Work out the finished part from the listing and answer in its coordinate system (mm). A direction names the side the tool comes from. Round coordinates to 2 decimals unless told otherwise and drop trailing zeros. Loops run counter-clockwise (first coordinate to the right, second up) from the corner with the lowest first, then second, coordinate; pieces in that order, holes last. Notation, with made-up numbers: (32.5, 81.5) - (79.5, 81.5) arc R19 cw to (79.5, 116.5) - close; hole circle Ø10 at (54.5, 34). An arc over 180 degrees is marked (long way). Use CSV: the item, a comma, the result in double quotes. Start each with the question number.
from build123d import *

# Parameters (mm, degrees)
ESQUISSE1_R                  = 4.15
BOSS_EXTRU_1_DEPTH           = 15
ENL_V_MAT_EXTRU_1_REACH      = 122
ENL_V_MAT_EXTRU_1_END_RADIUS = 4.15
ESQUISSE2_R                  = 4.15
ENL_V_MAT_EXTRU_2_DEPTH      = 7.5
TROU_TARAUD_M6X1_01_D        = 5


with BuildPart() as part:
    # Esquisse1 → Boss.-Extru.1 (new body)
    with BuildSketch(Plane(origin=(0, 0, 0), x_dir=(1, 0, 0), z_dir=(0, 1, 0))):
        with BuildLine():
            Line((25, 31.224989992), (25, 95))
            ThreePointArc((25, 95), (0, 120), (-25, 95))
            Line((-25, 95), (-25, 31.224989992))
            ThreePointArc((-25, 31.224989992), (0, 40), (25, 31.224989992))
        make_face()
        with Locations(Location((0, 95, 0), (0, 0, 270))):  # turned: the seam where the file's is
            Circle(ESQUISSE1_R, mode=Mode.SUBTRACT)
    extrude(amount=BOSS_EXTRU_1_DEPTH)

    # Enlèv. mat.-Extru.1: up to this cylinder (the profile starts outside it)
    enl_v_mat_extru_1_end = Plane(origin=(0, 7.5, -95), z_dir=(0, -1, 0)) * Cylinder(ENL_V_MAT_EXTRU_1_END_RADIUS, 253.3, mode=Mode.PRIVATE)
    # Esquisse2 → Enlèv. mat.-Extru.1 (cut, up to the surface)
    with BuildSketch(Plane.XY, mode=Mode.PRIVATE) as enl_v_mat_extru_1_sk1:
        with Locations((0, 7.5)):
            Circle(ESQUISSE2_R)
    enl_v_mat_extru_1_tool1 = extrude(enl_v_mat_extru_1_sk1.sketch, amount=-ENL_V_MAT_EXTRU_1_REACH, mode=Mode.PRIVATE) - enl_v_mat_extru_1_end
    add(enl_v_mat_extru_1_tool1.solids().sort_by_distance((0, 7.5, 0))[0], mode=Mode.SUBTRACT)

    # Esquisse3 → Enlèv. mat.-Extru.2 (cut)
    with BuildSketch(Plane(origin=(0, 15, 0), x_dir=(-1, 0, 0), z_dir=(0, 1, 0))):
        with BuildLine():
            Line((4.15, -95), (4.15, -86.15))
            ThreePointArc((4.15, -86.15), (0, -82), (-4.15, -86.15))
            Line((-4.15, -86.15), (-4.15, -95))
            ThreePointArc((-4.15, -95), (0, -99.15), (4.15, -95))
        make_face()
    extrude(amount=-ENL_V_MAT_EXTRU_2_DEPTH, mode=Mode.SUBTRACT)

    # Trou taraudé M6x1.01 (through all)
    with Locations(Plane.XZ):
        with Locations((17.5, -45), (-17.5, -45)):
            Hole(TROU_TARAUD_M6X1_01_D / 2)


solid = part.part
Item 1: Which of the six approach directions +Z, -Z, +X, -X, +Y, -Y give full straight-line access (tool end or side, diameter ignored) to faces 1 (the cylindrical face through (-0.9, 3.45, -60.87)), 2 (the flat face through (-4.15, 11, -91)), 3 (the cylindrical face through (0, 12, -40))?
Item 2: Find the intervals of material crossed by probe 1 along X at (y, z) = (6.5, -95); probe 2 along Z at (x, y) = (-17.5, 4); probe 3 along X at (y, z) = (8.5, -68), in increasing order. Write a range as [from, to].
Item 3: The mould has two halves that part along Z. Classify faces 4 (the cylindrical face through (-16, 8, -47)), 5 (the cylindrical face through (0.55, 7.395, -119.994)), 6 (the flat face through (4.15, 11, -91)), 7 (the flat face through (25, 7, -63)): pulls with the +Z half, pulls with the -Z half, needs draft (parallel to the pull), parting line crosses it, or undercut.
Item 4: A cutting plane is placed at A-A (z = -45). Determine the outline of the cut face in (x, y).
Item 5: A cutting plane is placed at D-D (y = 5). Determine the outline of the cut face in (x, z).
Item 6: A cutting plane is placed at C-C (y = 13.75). Determine the outline of the cut face in (x, z), plus the area to 3 significant figures.
Item 7: Each of these flat-tipped pins is pushed along its axis until it touches: pin 1 Ø2 at (x, y) = (15, 4) entering from -Z; pin 2 Ø8 at (x, y) = (-13, 10.5) entering from +Z; pin 3 Ø4 at (x, y) = (-18, 5.5) entering from -Z; pin 4 Ø8 at (x, z) = (-17.5, -45) entering from -Y. Where does it stop, or does it pass through?
Item 8: A cutting plane is placed at B-B (x = 0). Determine the outline of the cut face in (y, z).
Result sheet:
1,face 1,"+Z"
1,face 2,"+Y"
1,face 3,"+Z, +Y, -Y"
2,probe 1,"[-25, -4.15], [4.15, 25]"
2,probe 2,"[-112.85, -47.5], [-42.5, -35.97]"
2,probe 3,"[-25, -4.03], [4.03, 25]"
3,face 4,"undercut"
3,face 5,"pulls with the -Z half"
3,face 6,"undercut"
3,face 7,"needs draft"
4,outline,"(-25, 0) - (-20, 0) - (-20, 15) - (-25, 15) - close; (-15, 0) - (15, 0) - (15, 15) - (-15, 15) - close; (20, 0) - (25, 0) - (25, 15) - (20, 15) - close; hole circle Ø8.3 at (0, 7.5)"
5,outline,"(-25, -95) arc R25 ccw to (25, -95) - (25, -31.22) arc R40 cw to (3.31, -39.86) - (3.31, -92.5) arc R4.15 cw (long way) to (-3.31, -92.5) - (-3.31, -39.86) arc R40 cw to (-25, -31.22) - close; hole circle Ø5 at (-17.5, -45); hole circle Ø5 at (17.5, -45)"
6,outline,"(-25, -95) arc R25 ccw to (25, -95) - (25, -31.22) arc R40 cw to (-25, -31.22) - close; hole circle Ø5 at (-17.5, -45); hole (-4.15, -95) arc R4.15 ccw to (4.15, -95) - (4.15, -86.15) arc R4.15 ccw to (-4.15, -86.15) - close; hole circle Ø5 at (17.5, -45)"
6,area,"3,700 mm^2"
7,pin 1,"z = -115.71"
7,pin 2,"z = -36.21"
7,pin 3,"z = -114.21"
7,pin 4,"y = 0"
8,outline,"(0, -120) - (15, -120) - (15, -99.15) - (0, -99.15) - close; (0, -90.85) - (3.35, -90.85) - (3.35, -40) - (0, -40) - close; (11.65, -82) - (15, -82) - (15, -40) - (11.65, -40) - close"
